```python
from build123d import *

# Parameters (mm, degrees)
CYLINDER002_R     = 0.875
CYLINDER002_DEPTH = 10
EXTRUDE_DEPTH     = 1.59


with BuildPart() as cylinder002:
    # Cylinder002 → Cylinder002 (new body)
    with BuildSketch(Plane.XY):
        Circle(CYLINDER002_R)
    extrude(amount=CYLINDER002_DEPTH)


with BuildPart() as cut017:
    # InvoluteGear → Extrude (new body)
    with BuildSketch(Plane.XY):
        with BuildLine():
            Line((2.145433, -0.523441), (2.728817, -0.664878))
            add(Edge.make_bspline(
                [(2.728817, -0.664878), (2.761585, -0.669616), (2.859596, -0.677652), (3.02783, -0.638771)],
                knots=[0, 0, 0, 0, 1, 1, 1, 1], degree=3))
            add(Edge.make_bspline(
                [(3.02783, -0.638771), (3.226212, -0.590574), (3.503888, -0.476829), (3.820611, -0.215776)],
                knots=[0, 0, 0, 0, 1, 1, 1, 1], degree=3))
            ThreePointArc((3.820611, -0.215776), (3.826702, 0), (3.820611, 0.215776))
            add(Edge.make_bspline(
                [(3.820611, 0.215776), (3.503888, 0.476829), (3.226212, 0.590574), (3.02783, 0.638771)],
                knots=[0, 0, 0, 0, 1, 1, 1, 1], degree=3))
            add(Edge.make_bspline(
                [(3.02783, 0.638771), (2.859596, 0.677652), (2.761585, 0.669616), (2.728817, 0.664878)],
                knots=[0, 0, 0, 0, 1, 1, 1, 1], degree=3))
            Line((2.728817, 0.664878), (2.145433, 0.523441))
            ThreePointArc((2.145433, 0.523441), (1.925498, 0.548923), (1.775218, 0.711518))
            ThreePointArc((1.775218, 0.711518), (1.723103, 0.829803), (1.663117, 0.944297))
            ThreePointArc((1.663117, 0.944297), (1.629693, 1.163167), (1.746898, 1.351007))
            Line((1.746898, 1.351007), (2.221212, 1.718931))
            add(Edge.make_bspline(
                [(2.221212, 1.718931), (2.245347, 1.741595), (2.312739, 1.813213), (2.387233, 1.968986)],
                knots=[0, 0, 0, 0, 1, 1, 1, 1], degree=3))
            add(Edge.make_bspline(
                [(2.387233, 1.968986), (2.473239, 2.154137), (2.557438, 2.442152), (2.550813, 2.85254)],
                knots=[0, 0, 0, 0, 1, 1, 1, 1], degree=3))
            ThreePointArc((2.550813, 2.85254), (2.38591, 2.991836), (2.213412, 3.121609))
            add(Edge.make_bspline(
                [(2.213412, 3.121609), (1.811838, 3.036748), (1.549781, 2.89057), (1.38841, 2.76552)],
                knots=[0, 0, 0, 0, 1, 1, 1, 1], degree=3))
            add(Edge.make_bspline(
                [(1.38841, 2.76552), (1.253119, 2.658231), (1.198293, 2.576592), (1.181567, 2.54802)],
                knots=[0, 0, 0, 0, 1, 1, 1, 1], degree=3))
            Line((1.181567, 2.54802), (0.928413, 2.003727))
            ThreePointArc((0.928413, 2.003727), (0.771363, 1.847662), (0.550543, 1.831545))
            ThreePointArc((0.550543, 1.831545), (0.425571, 1.86455), (0.298655, 1.889037))
            ThreePointArc((0.298655, 1.889037), (0.106697, 1.999368), (0.032913, 2.20812))
            Line((0.032913, 2.20812), (0.040989, 2.808349))
            add(Edge.make_bspline(
                [(0.040989, 2.808349), (0.038317, 2.84135), (0.024342, 2.938692), (-0.051, 3.094056)],
                knots=[0, 0, 0, 0, 1, 1, 1, 1], degree=3))
            add(Edge.make_bspline(
                [(-0.051, 3.094056), (-0.142133, 3.276739), (-0.314814, 3.522142), (-0.6398, 3.772835)],
                knots=[0, 0, 0, 0, 1, 1, 1, 1], degree=3))
            ThreePointArc((-0.6398, 3.772835), (-0.851521, 3.730759), (-1.060532, 3.676806))
            add(Edge.make_bspline(
                [(-1.060532, 3.676806), (-1.244562, 3.309933), (-1.293666, 3.013909), (-1.296511, 2.809776)],
                knots=[0, 0, 0, 0, 1, 1, 1, 1], degree=3))
            add(Edge.make_bspline(
                [(-1.296511, 2.809776), (-1.296982, 2.637108), (-1.267337, 2.543343), (-1.255427, 2.512451)],
                knots=[0, 0, 0, 0, 1, 1, 1, 1], degree=3))
            Line((-1.255427, 2.512451), (-0.987721, 1.975166))
            ThreePointArc((-0.987721, 1.975166), (-0.963624, 1.755075), (-1.088702, 1.572382))
            ThreePointArc((-1.088702, 1.572382), (-1.192424, 1.495253), (-1.2907, 1.411294))
            ThreePointArc((-1.2907, 1.411294), (-1.496645, 1.330005), (-1.705856, 1.402472))
            Line((-1.705856, 1.402472), (-2.1701, 1.783023))
            add(Edge.make_bspline(
                [(-2.1701, 1.783023), (-2.197567, 1.80151), (-2.282385, 1.851276), (-2.450828, 1.889239)],
                knots=[0, 0, 0, 0, 1, 1, 1, 1], degree=3))
            add(Edge.make_bspline(
                [(-2.450828, 1.889239), (-2.650476, 1.931889), (-2.950005, 1.949888), (-3.34863, 1.852109)],
                knots=[0, 0, 0, 0, 1, 1, 1, 1], degree=3))
            ThreePointArc((-3.34863, 1.852109), (-3.44774, 1.660344), (-3.535874, 1.463293))
            add(Edge.make_bspline(
                [(-3.535874, 1.463293), (-3.363782, 1.090672), (-3.162956, 0.867712), (-3.005133, 0.738213)],
                knots=[0, 0, 0, 0, 1, 1, 1, 1], degree=3))
            add(Edge.make_bspline(
                [(-3.005133, 0.738213), (-2.870429, 0.630189), (-2.778637, 0.594904), (-2.747059, 0.584955)],
                knots=[0, 0, 0, 0, 1, 1, 1, 1], degree=3))
            Line((-2.747059, 0.584955), (-2.160081, 0.459265))
            ThreePointArc((-2.160081, 0.459265), (-1.972982, 0.34088), (-1.908132, 0.129183))
            ThreePointArc((-1.908132, 0.129183), (-1.9125, 0), (-1.908132, -0.129183))
            ThreePointArc((-1.908132, -0.129183), (-1.972982, -0.34088), (-2.160081, -0.459265))
            Line((-2.160081, -0.459265), (-2.747059, -0.584955))
            add(Edge.make_bspline(
                [(-2.747059, -0.584955), (-2.778637, -0.594904), (-2.870429, -0.630189), (-3.005133, -0.738213)],
                knots=[0, 0, 0, 0, 1, 1, 1, 1], degree=3))
            add(Edge.make_bspline(
                [(-3.005133, -0.738213), (-3.162956, -0.867712), (-3.363782, -1.090672), (-3.535874, -1.463293)],
                knots=[0, 0, 0, 0, 1, 1, 1, 1], degree=3))
            ThreePointArc((-3.535874, -1.463293), (-3.44774, -1.660344), (-3.34863, -1.852109))
            add(Edge.make_bspline(
                [(-3.34863, -1.852109), (-2.950005, -1.949888), (-2.650476, -1.931889), (-2.450828, -1.889239)],
                knots=[0, 0, 0, 0, 1, 1, 1, 1], degree=3))
            add(Edge.make_bspline(
                [(-2.450828, -1.889239), (-2.282385, -1.851276), (-2.197567, -1.80151), (-2.1701, -1.783023)],
                knots=[0, 0, 0, 0, 1, 1, 1, 1], degree=3))
            Line((-2.1701, -1.783023), (-1.705856, -1.402472))
            ThreePointArc((-1.705856, -1.402472), (-1.496645, -1.330005), (-1.2907, -1.411294))
            ThreePointArc((-1.2907, -1.411294), (-1.192424, -1.495253), (-1.088702, -1.572382))
            ThreePointArc((-1.088702, -1.572382), (-0.963624, -1.755075), (-0.987721, -1.975166))
            Line((-0.987721, -1.975166), (-1.255427, -2.512451))
            add(Edge.make_bspline(
                [(-1.255427, -2.512451), (-1.267337, -2.543343), (-1.296982, -2.637108), (-1.296511, -2.809776)],
                knots=[0, 0, 0, 0, 1, 1, 1, 1], degree=3))
            add(Edge.make_bspline(
                [(-1.296511, -2.809776), (-1.293666, -3.013909), (-1.244562, -3.309933), (-1.060532, -3.676806)],
                knots=[0, 0, 0, 0, 1, 1, 1, 1], degree=3))
            ThreePointArc((-1.060532, -3.676806), (-0.851521, -3.730759), (-0.6398, -3.772835))
            add(Edge.make_bspline(
                [(-0.6398, -3.772835), (-0.314814, -3.522142), (-0.142133, -3.276739), (-0.051, -3.094056)],
                knots=[0, 0, 0, 0, 1, 1, 1, 1], degree=3))
            add(Edge.make_bspline(
                [(-0.051, -3.094056), (0.024342, -2.938692), (0.038317, -2.84135), (0.040989, -2.808349)],
                knots=[0, 0, 0, 0, 1, 1, 1, 1], degree=3))
            Line((0.040989, -2.808349), (0.032913, -2.20812))
            ThreePointArc((0.032913, -2.20812), (0.106697, -1.999368), (0.298655, -1.889037))
            ThreePointArc((0.298655, -1.889037), (0.425571, -1.86455), (0.550543, -1.831545))
            ThreePointArc((0.550543, -1.831545), (0.771363, -1.847662), (0.928413, -2.003727))
            Line((0.928413, -2.003727), (1.181567, -2.54802))
            add(Edge.make_bspline(
                [(1.181567, -2.54802), (1.198293, -2.576592), (1.253119, -2.658231), (1.38841, -2.76552)],
                knots=[0, 0, 0, 0, 1, 1, 1, 1], degree=3))
            add(Edge.make_bspline(
                [(1.38841, -2.76552), (1.549781, -2.89057), (1.811838, -3.036748), (2.213412, -3.121609)],
                knots=[0, 0, 0, 0, 1, 1, 1, 1], degree=3))
            ThreePointArc((2.213412, -3.121609), (2.38591, -2.991836), (2.550813, -2.85254))
            add(Edge.make_bspline(
                [(2.550813, -2.85254), (2.557438, -2.442152), (2.473239, -2.154137), (2.387233, -1.968986)],
                knots=[0, 0, 0, 0, 1, 1, 1, 1], degree=3))
            add(Edge.make_bspline(
                [(2.387233, -1.968986), (2.312739, -1.813213), (2.245347, -1.741595), (2.221212, -1.718931)],
                knots=[0, 0, 0, 0, 1, 1, 1, 1], degree=3))
            Line((2.221212, -1.718931), (1.746898, -1.351007))
            ThreePointArc((1.746898, -1.351007), (1.629693, -1.163167), (1.663117, -0.944297))
            ThreePointArc((1.663117, -0.944297), (1.723103, -0.829803), (1.775218, -0.711518))
            ThreePointArc((1.775218, -0.711518), (1.925498, -0.548923), (2.145433, -0.523441))
        make_face()
    extrude(amount=EXTRUDE_DEPTH)

    # Cut017: cut Cylinder002
    add(cylinder002.part, mode=Mode.SUBTRACT)


solid = cut017.part
```
The listing builds one solid part. Answer for the finished solid, in the listing's coordinates (mm). Round coordinates to 2 decimals unless told otherwise and drop trailing zeros. Order: outer loops, then holes, each group sorted by start corner. A loop starts at its lowest first (then second) coordinate and runs counter-clockwise, first axis right, second up. Notation, with made-up numbers: (86, -16) - (90, -16) arc R23 ccw to (90, -7) - close; hole circle Ø6 at (-16.5, 15.25). An arc over 180 degrees is marked (long way). Put each result on its own line as item: value. Start each with the question number.
(1) Find section A-A (y = 0). Give the vertices of the cut face in (x, z) (1 decimal).
(2) Find section C-C (x = 2). State how many separate pieces and enclosed holes the cut face has, plus the area to 3 significant figures.
(3) Determine the mould class of faces 1 (the flat face through (-1, 1, 0)), 2 (the cylindrical face through (0.808, -0.335, 0.784)) for opening direction Y: released by +Y, released by -Y, zero draft, split by the parting line, or undercut.
(4) Straight lines are drawn through the part: probe 1 along Y at (x, z) = (2.75, 0.5); probe 2 along X at (y, z) = (-0.25, 0.5); probe 3 along Y at (x, z) = (-3, 0.4). For each, find the intervals that lie inside material, in ascending order. Write a range as from..to.
(5) Find section B-B (x = -0.75). Give the vertices of the cut face in (y, z).
Reply:
1. outline: (-1.9, 0) - (-0.9, 0) - (-0.9, 1.6) - (-1.9, 1.6) - close; (0.9, 0) - (3.8, 0) - (3.8, 1.6) - (0.9, 1.6) - close
2. separate pieces: 3
2. enclosed holes: 0
2. area: 6.49 mm^2
3. face 1: zero draft
3. face 2: undercut
4. probe 1: -0.67..0.67
4. probe 2: -1.92..-0.84, 0.84..3.78
4. probe 3: -1.91..-0.73, 0.73..1.91
5. outline: (-3.75, 0) - (-0.45, 0) - (-0.45, 1.59) - (-3.75, 1.59) - close; (0.45, 0) - (3.75, 0) - (3.75, 1.59) - (0.45, 1.59) - close
